from build123d import *

# Parameters (mm, degrees)
BOSS_EXTRUDE1_DEPTH = 6.35
BOSS_EXTRUDE2_START = 50.8
BOSS_EXTRUDE2_DEPTH = 50.8
LPATTERN1_COUNT     = 2
LPATTERN1_PITCH     = 50.8
BOSS_EXTRUDE3_DEPTH = 6.35


with BuildPart() as part:
    # Sketch1 → Boss-Extrude1 (new, symmetric)
    with BuildSketch(Plane.XY):
        with BuildLine():
            Line((3.2766, 0), (3.2766, -85.725))
            ThreePointArc((3.2766, -85.725), (4.5466, -86.995), (5.8166, -85.725))
            Line((5.8166, -85.725), (5.8166, 0))
            ThreePointArc((5.8166, 0), (-1.258942658, 5.678723355), (-5.271629874, -2.458201381))
            ThreePointArc((-5.271629874, -2.458201381), (-3.583893792, -3.072487078), (-2.969608095, -1.384750996))
            ThreePointArc((-2.969608095, -1.384750996), (-0.709186039, 3.198931497), (3.2766, 0))
        make_face()
    boss_extrude1 = extrude(amount=BOSS_EXTRUDE1_DEPTH, both=True)

    # Sketch2 → Boss-Extrude2 (add)
    with BuildSketch(Plane.XY.offset(6.35).offset(BOSS_EXTRUDE2_START)):
        with BuildLine():
            Line((3.2766, 0), (5.8166, 0))
            Line((5.8166, 0), (5.8166, -85.725))
            ThreePointArc((5.8166, -85.725), (4.5466, -86.995), (3.2766, -85.725))
            Line((3.2766, -85.725), (3.2766, 0))
        make_face()
    extrude(amount=-BOSS_EXTRUDE2_DEPTH)

    # LPattern1: Boss-Extrude1 ×2
    with Locations(*[(0, 0, i * LPATTERN1_PITCH) for i in range(1, LPATTERN1_COUNT)]):
        add(boss_extrude1)

    # Sketch4 → Boss-Extrude3 (add, symmetric)
    with BuildSketch(Plane.XY.offset(25.4)):
        with BuildLine():
            Line((3.2766, -66.802), (3.2766, -71.607905534))
            ThreePointArc((3.2766, -71.607905534), (-3.956296051, -71.065866451), (-5.037323364, -63.8937))
            Line((-5.037323364, -63.8937), (-2.837618838, -65.1637))
            ThreePointArc((-2.837618838, -65.1637), (-0.848046483, -69.966952562), (3.2766, -66.802))
        make_face()
    extrude(amount=BOSS_EXTRUDE3_DEPTH, both=True)


solid = part.part
Part model, mm, in its own coordinate system. A direction names the side the tool comes from. Give positions to 0.01 mm unless a question says otherwise; leave off trailing zeros. Order: outer loops, then holes, each group sorted by start corner. A loop starts at its lowest first (then second) coordinate and runs counter-clockwise, first axis right, second up. Notation, with made-up numbers: (23.25, 27) - (66.25, 27) arc R34 ccw to (66.25, 58) - close; hole circle Ø7 at (28, -27). An arc over 180 degrees is marked (long way). Use a Markdown table: item, result.
1) Saw through at D-D on z = 9. List the corners of the cut face in (x, y) (3 decimals), plus the area to 3 significant figures.
Checked values:
| item | result |
|---|---|
| outline | (3.277, -85.725) arc R1.27 ccw to (5.817, -85.725) - (5.817, 0) - (3.277, 0) - close |
| area | 220 mm² |
2) Flat gauge pins, fed straight in: P1, Ø4, axis at y = -46, z = 7, coming from the -X side; P2, Ø2.5, axis at x = -1.5, y = -69, coming from the +Z side; P3, Ø1.5, axis at x = 3, z = 3, coming from the +Y side; P4, Ø5, axis at x = 0, y = -66.802, coming from the +Z side. Where does each tip first touch, or does it go through?
Checked values:
| item | result |
|---|---|
| P1 | x = 3.28 |
| P2 | z = 31.75 |
| P3 | y = 5.36 |
| P4 | through |
3) 3-axis set-ups, long thin cutter, end or side, ignore diameter. For faces 4 (the flat face through (-2, -70, 19.05)), 5 (the cylindrical face through (4.575, -86.995, 25.844)), 6 (the flat face through (-2, -70, 31.75)), 7 (the flat face through (5, 0, 26)), 8 (the flat face through (-1.4, 3.4, 44.45)): which of +Z, -Z, +X, -X, +Y, -Y reach the whole face in a straight line?
Checked values:
| item | result |
|---|---|
| face 4 | -Z, -X, +Y, -Y |
| face 5 | +Z, -Z, -Y |
| face 6 | +Z, -X, +Y, -Y |
| face 7 | +X, -X, +Y |
| face 8 | -X, +Y |
4) Saw through at B-B on y = -17.5. List the corners of the cut face in (x, z).
Checked values:
| item | result |
|---|---|
| outline | (3.28, -6.35) - (5.82, -6.35) - (5.82, 57.15) - (3.28, 57.15) - close |
5) Probe L1, parallel to X at y = 0, z = 2; L2, parallel to Y at x = 0, z = 22.5; L3, parallel to X at y = -79, z = 4.5. List the from-to ranges inside material, lowest first. Write a range as from..to.
Checked values:
| item | result |
|---|---|
| L1 | -5.82..-3.28, 3.28..5.82 |
| L2 | -72.62..-70.08 |
| L3 | 3.28..5.82 |
6) Saw through at A-A on x = 0. List the corners of the cut face in (y, z).
Checked values:
| item | result |
|---|---|
| outline | (-72.62, 19.05) - (-70.08, 19.05) - (-70.08, 31.75) - (-72.62, 31.75) - close; (3.28, -6.35) - (5.82, -6.35) - (5.82, 6.35) - (3.28, 6.35) - close; (3.28, 44.45) - (5.82, 44.45) - (5.82, 57.15) - (3.28, 57.15) - close |
7) Saw through at C-C on z = 48. List the corners of the cut face in (x, y) (3 decimals), plus the area to 3 significant figures.
Checked values:
| item | result |
|---|---|
| outline | (-5.272, -2.458) arc R1.27 ccw to (-2.97, -1.385) arc R3.277 cw (long way) to (3.277, 0) - (3.277, -85.725) arc R1.27 ccw to (5.817, -85.725) - (5.817, 0) arc R5.817 ccw (long way) to start |
| area | 264 mm² |
8) Two-plate mould, pull along Y, no slides. Class faces 1 (the cylindrical face through (-0.79, 3.18, 50.89)), 2 (the flat face through (3.5, -36.9, 57.15)), 3 (the flat face through (-3.95, -64.52, 25.49)): +Y half, -Y half, draft (parallel to the pull), parting line (faces both ways), or undercut.
Checked values:
| item | result |
|---|---|
| face 1 | undercut |
| face 2 | draft |
| face 3 | +Y half |
